Can you work these out from the model? Positions are in its coordinate system, mm. A direction names the side the tool comes from. Give positions to 0.01 mm unless a question says otherwise; leave off trailing zeros. Loops run counter-clockwise (first coordinate to the right, second up) from the corner with the lowest first, then second, coordinate; pieces in that order, holes last. Notation, with made-up numbers: (-34, -36.5) - (2, -36.5) arc R25 cw to (2, -11.5) - close; hole circle Ø9 at (89, 17). An arc over 180 degrees is marked (long way). Write item = value, one per line.
from build123d import *

# Parameters (mm, degrees)
SKETCH1_W           = 88.9
SKETCH1_H           = 31.75
BOSS_EXTRUDE1_DEPTH = 12.7
SKETCH2_R           = 4.7625
BOSS_EXTRUDE2_DEPTH = 57.15


with BuildPart() as part:
    # Sketch1 → Boss-Extrude1 (new body)
    with BuildSketch(Plane(origin=(0, 0, 0), x_dir=(1, 0, 0), z_dir=(0, 1, 0))):
        Rectangle(SKETCH1_W, SKETCH1_H)
    extrude(amount=BOSS_EXTRUDE1_DEPTH)

    # Sketch2 → Boss-Extrude2 (add)
    with BuildSketch(Plane.ZY.offset(44.45)):
        with Locations((0, 6.35)):
            Circle(SKETCH2_R)
    extrude(amount=BOSS_EXTRUDE2_DEPTH)


solid = part.part
Q1. For pin 1 (5 mm diameter, centred on x = -81.5, z = 7.5, fed in from -Y); pin 2 (6 mm diameter, centred on y = 7, z = 10.5, fed in from -X), each with a flat end and sliding along its axis, tell me the tip position at first contact or that it passes through.
Output:
pin_1 = through
pin_2 = -44.45
Q2. Imagine slicing it at A-A, the plane z = 1. Write out the boundary of the cut face in (x, y).
Output:
outline = (-101.6, 1.69) - (-44.45, 1.69) - (-44.45, 0) - (44.45, 0) - (44.45, 12.7) - (-44.45, 12.7) - (-44.45, 11.01) - (-101.6, 11.01) - close
Q3. Imagine slicing it at C-C, the plane z = -12. Write out the boundary of the cut face in (x, y).
Output:
outline = (-44.45, 0) - (44.45, 0) - (44.45, 12.7) - (-44.45, 12.7) - close
Q4. Imagine slicing it at B-B, the plane y = 3.5. Write out the boundary of the cut face in (x, z) (3 decimals), then the cut area to 3 significant figures.
Output:
outline = (-101.6, -3.816) - (-44.45, -3.816) - (-44.45, -15.875) - (44.45, -15.875) - (44.45, 15.875) - (-44.45, 15.875) - (-44.45, 3.816) - (-101.6, 3.816) - close
area = 3,260 mm2
Q5. Which directions (+Z, -Z, +X, -X, +Y, -Y) give clear straight access to the entire face, cutting with the end or side of a thin tool? Please do faces 1 (the cylindrical face through (-72.62, 1.7, -1.03)), 2 (the flat face through (-1, 12.7, 0)).
Output:
face_1 = -X
face_2 = +Z, -Z, +X, -X, +Y
Q6. I need wall thicknesses on L1, parallel to X at y = 3.25, z = 13; L2, parallel to Y at x = -79.5, z = -3; L3, parallel to Z at x = -90.5, y = 5. Which ranges of each line are inside material? Lowest first, please.
Output:
L1 = -44.45 to 44.45
L2 = 2.65 to 10.05
L3 = -4.57 to 4.57
